Read the model definition and answer for the solid it produces. Units are mm, in the model's axes. A direction names the side the tool comes from. Coordinates: 2 decimals unless noted, no trailing zeros. Write each loop counter-clockwise with the first axis right and the second up, starting at its lowest first coordinate (ties: lowest second). Pieces come first, ordered by that corner, then holes. Notation, with made-up numbers: M 76.25,-8.75 L 123.25,-8.75 A20 cw 123.25,13.25 Z; hole C -13.75,72 d11. An arc over 180 degrees is marked long. Write item = value, one per line.
from build123d import *

# Parameters (mm, degrees)
REVOLVE1_ANGLE      = 57
BOSS_EXTRUDE1_DEPTH = 25.4
SKETCH8_R           = 152.4
CUT_EXTRUDE3_DEPTH  = 257.048
SKETCH13_W          = 16.387620484
SKETCH13_H          = 127
CUT_EXTRUDE5_DEPTH  = 1.778
BOSS_EXTRUDE3_DEPTH = 25.4


with BuildPart() as part:
    # Sketch1 → Revolve1 (revolve)
    with BuildSketch(Plane.XY):
        with BuildLine():
            Line((-59.991213716, 144.035687339), (-8.193810242, 180.296949153))
            ThreePointArc((-8.193810242, 180.296949153), (0, 182.88), (8.193810242, 180.296949153))
            Line((8.193810242, 180.296949153), (59.991213716, 144.035687339))
            add(Edge.make_bspline(
                [(59.991213716, 144.035687339), (62.78248672, 142.0840471), (62.441206007, 139.021062406)],
                knots=[0, 0, 0, 1, 1, 1], degree=2))
            ThreePointArc((62.441206007, 139.021062406), (0, 152.4), (-62.441206007, 139.021062406))
            add(Edge.make_bspline(
                [(-59.991213716, 144.035687339), (-62.78248672, 142.0840471), (-62.441206007, 139.021062406)],
                knots=[0, 0, 0, 1, 1, 1], degree=2))
        make_face()
    revolve(axis=Axis((0, 0, 0), (-1, 0, 0)), revolution_arc=REVOLVE1_ANGLE)

    # Sketch3 → Boss-Extrude1 (add)
    with BuildSketch(Plane.XY):
        with BuildLine():
            Line((-59.991213716, 144.035687339), (-8.193810242, 180.296949153))
            ThreePointArc((-8.193810242, 180.296949153), (0, 182.88), (8.193810242, 180.296949153))
            Line((8.193810242, 180.296949153), (59.991213716, 144.035687339))
            add(Edge.make_bspline(
                [(59.991213716, 144.035687339), (62.782486262, 142.084047002), (62.441206007, 139.021062406)],
                knots=[0, 0, 0, 1, 1, 1], degree=2))
            ThreePointArc((62.441206007, 139.021062406), (0, 152.4), (-62.441206007, 139.021062406))
            add(Edge.make_bspline(
                [(-59.991213716, 144.035687339), (-62.782486262, 142.084047002), (-62.441206007, 139.021062406)],
                knots=[0, 0, 0, 1, 1, 1], degree=2))
        make_face()
    extrude(amount=BOSS_EXTRUDE1_DEPTH)

    # Sketch7 → Cut-Revolve2 (revolve, cut)
    with BuildSketch(Plane.XY.offset(12.7)):
        Polygon((-18.85509192, 148.029004366), (-21.456080621, 146.208157646), (-33.109499632, 162.854485329), (-27.584999632, 166.721963764), (-28.163260355, 161.325258604), align=None)
    cut_revolve2 = revolve(axis=Axis((-21.456080621, 146.208157646, 12.7), (-0.57349503, 0.81920904, 0)), mode=Mode.SUBTRACT)

    # Mirror2: Cut-Revolve2 across plane
    add(cut_revolve2.mirror(Plane(origin=(0, 0, 0), x_dir=(0, 0, 1), z_dir=(1, 0, 0))), mode=Mode.SUBTRACT)

    # Sketch8 → Cut-Extrude3 (cut)
    with BuildSketch(Plane.XY.offset(25.4)):
        Circle(SKETCH8_R)
    extrude(amount=-CUT_EXTRUDE3_DEPTH, mode=Mode.SUBTRACT)

    # Sketch13 → Cut-Extrude5 (cut)
    with BuildSketch(Plane(origin=(0, 167.069193294, -74.383997286), x_dir=(1, 0, 0), z_dir=(0, 0.913545458, -0.406736643))):
        Rectangle(SKETCH13_W, SKETCH13_H)
    extrude(amount=-CUT_EXTRUDE5_DEPTH, mode=Mode.SUBTRACT)

    # Sketch14 → Cut-Revolve4 (revolve, cut)
    with BuildSketch(Plane(origin=(0, 0, 0), x_dir=(0, 0, -1), z_dir=(1, 0, 0))):
        Polygon((73.660819534, 165.44490947), (67.500143032, 168.18781937), (69.097003878, 163.000445517), (60.429201972, 143.532243688), (63.3297088, 142.240854846), align=None)
    revolve(axis=Axis((0, 165.44490947, -73.660819534), (0, -0.913545458, 0.406736643)), mode=Mode.SUBTRACT)

    # Sketch15 → Boss-Extrude3 (add)
    with BuildSketch(Plane.XY.offset(25.4)):
        with BuildLine():
            Line((-11.1125, 168.5925), (-11.1125, 151.994316814))
            ThreePointArc((-11.1125, 151.994316814), (-8.732319534, 152.149619111), (-6.35, 152.267650865))
            Line((-6.35, 152.267650865), (-6.35, 168.5925))
            ThreePointArc((-6.35, 168.5925), (0, 174.9425), (6.35, 168.5925))
            Line((6.35, 168.5925), (6.35, 152.267650865))
            ThreePointArc((6.35, 152.267650865), (8.732319534, 152.149619111), (11.1125, 151.994316814))
            Line((11.1125, 151.994316814), (11.1125, 168.5925))
            ThreePointArc((11.1125, 168.5925), (0, 179.705), (-11.1125, 168.5925))
        make_face()
    extrude(amount=BOSS_EXTRUDE3_DEPTH)


solid = part.part
Item 1: Find section A-A (x = 0). Determine the outline of the cut face in (y, z) (1 decimal).
Worked answers:
outline = M 152.4,-101.1 A182.9 ccw 155.1,-96.9 L 162.7,-79.8 L 160.4,-74.9 L 152.4,-71.3 Z; M 152.4,-64.4 L 163,-69.1 L 168.2,-67.5 L 175.8,-50.4 A182.9 ccw 182.9,0 L 182.9,25.4 L 179.7,25.4 L 179.7,50.8 L 174.9,50.8 L 174.9,25.4 L 152.4,25.4 Z
Item 2: Find section B-B (x = -54). Determine the outline of the cut face in (y, z).
Worked answers:
outline = M 142.51,-40.77 A148.23 ccw 148.23,0 L 148.23,25.4 L 142.51,25.4 Z
Item 3: Which of the six approach directions +Z, -Z, +X, -X, +Y, -Y give full straight-line access (tool end or side, diameter ignored) to faces 4 (the face through (6.35, 161, 38)), 5 (the face through (-11.112, 160, 38)), 6 (the face through (11.112, 160, 38))?
Worked answers:
face_4 = +Z, -Y
face_5 = +Z, -X, +Y, -Y
face_6 = +Z, +X, +Y, -Y
Item 4: For a pull along Z with two mould halves and no side action, classify faces 1 (the face through (14, 159, 25.4)), 2 (the face through (39.49, 158.39, 12.52)), 3 (the face through (-2.82, 162.62, -70.43)) as released by +Z, released by -Z, zero draft, split by the parting line, or undercut.
Worked answers:
face_1 = released by +Z
face_2 = zero draft
face_3 = undercut
Item 5: Find section C-C (x = 45.5). Determine the outline of the cut face in (y, z).
Worked answers:
outline = M 145.45,-51.15 A154.18 ccw 154.18,0 L 154.18,25.4 L 145.45,25.4 Z
Item 6: Flat-ended cylindrical pins translate along their axes: pin 1 (8 mm diameter, centred on y = 164, z = 32, fed in from +X); pin 2 (4 mm diameter, centred on x = 3, y = 166.5, fed in from +Z); pin 3 (13 mm diameter, centred on y = 163, z = 38.5, fed in from -X). Find the tip coordinate at first contact, or state that the pin passes through.
Worked answers:
pin_1 = 11.11
pin_2 = 25.4
pin_3 = -11.11
Item 7: Consider line 1 along X through (y, z) = (165, -70); line 2 along Y through (x, z) = (14, -75.5); line 3 along Y through (x, z) = (-54.5, -24). Determine where each line is inside the solid, lowest interval first. Write a range as from..to.
Worked answers:
line_1 = -9.71..-3.99, 3.99..9.71
line_2 = 151.76..159.24
line_3 = 142.32..145.92
